Work out the finished part from the listing and answer in its coordinate system (mm). A direction names the side the tool comes from. Coordinates: 2 decimals unless noted, no trailing zeros. Loops run counter-clockwise (first coordinate to the right, second up) from the corner with the lowest first, then second, coordinate; pieces in that order, holes last. Notation, with made-up numbers: (-26, 13.5) -> (11, 13.5) arc R14 cw to (11, 28.5) -> close; hole circle Ø2 at (40.25, 76.5). An arc over 180 degrees is marked (long way). Use a Markdown table: item, result.
from build123d import *

# Parameters (mm, degrees)
F1_DEPTH = 50.8
F0_R     = 1.016
F2_DEPTH = 31.496
F3_R     = 2.159
F4_DEPTH = 20.32
F3_W     = 39.116
F3_H     = 6.35
F3_H_2   = 9.431579427
F5_DEPTH = 25.4
F6_W     = 95.504
F6_H     = 27.8849071284
F7_DEPTH = 35.56


with BuildPart() as f1:
    # F0 (on Right) → F1 (new body, symmetric)
    with BuildSketch(Plane.YZ):
        Polygon((-42.0039315899, 10.0997092374), (-35.6157857536, 10.0997092374), (8.7960684101, 10.0997092374), (6.0031614266, 16.4607279003), (-42.0039315899, 35.4997092374), (-42.0039315899, 20.2597092374), align=None)
    extrude(amount=F1_DEPTH, both=True)

    # F0 (on Right) → F2 (join, symmetric)
    with BuildSketch(Plane.YZ):
        with BuildLine():
            Line((-48.3539315899, 10.0997092374), (-42.0039315899, 10.0997092374))
            Line((-42.0039315899, 10.0997092374), (-42.0039315899, 20.2597092374))
            Line((-42.0039315899, 20.2597092374), (-48.3539315899, 20.2597092374))
            ThreePointArc((-48.3539315899, 20.2597092374), (-51.0480084262, 19.1437860737), (-52.1639315899, 16.4497092374))
            Line((-52.1639315899, 16.4497092374), (-52.1639315899, 13.9097092374))
            ThreePointArc((-52.1639315899, 13.9097092374), (-51.0480084262, 11.215632401), (-48.3539315899, 10.0997092374))
        make_face()
        with Locations((-47.7287806571, 15.2929993346)):
            Circle(F0_R, mode=Mode.SUBTRACT)
    extrude(amount=F2_DEPTH, both=True)

    # F3 (on face) → F4 (join)
    with BuildSketch(Plane.XY.offset(20.2597092374)):
        with Locations((-24.638, -45.1789315899)):
            Circle(F3_R)
        with Locations((24.638, -45.1789315899)):
            Circle(F3_R)
    extrude(amount=F4_DEPTH)

    # F3 (on face) → F5 (cut)
    with BuildSketch(Plane.XY.offset(20.2597092374)):
        with Locations((0, -45.1789315899)):
            Rectangle(F3_W, F3_H)
        with Locations((0, -53.0697213034)):
            Rectangle(F3_W, F3_H_2)
    extrude(amount=-F5_DEPTH, mode=Mode.SUBTRACT)

    # F6 (on Front) → F7 (cut, symmetric)
    with BuildSketch(Plane.XZ):
        with Locations((0, 27.0901628016)):
            Rectangle(F6_W, F6_H)
    extrude(amount=F7_DEPTH, both=True, mode=Mode.SUBTRACT)


solid = f1.part
Q1. Section D-D on x = -24 is taken. Determine the outline of the cut face in (y, z), and give its area (3 significant figures).
Solved:
| item | result |
|---|---|
| outline | (-52.16, 13.91) arc R3.81 ccw to (-48.35, 10.1) -> (8.8, 10.1) -> (7.46, 13.15) -> (-35.56, 13.15) -> (-35.56, 32.94) -> (-42, 35.5) -> (-42, 20.26) -> (-43.12, 20.26) -> (-43.12, 40.58) -> (-47.24, 40.58) -> (-47.24, 20.26) -> (-48.35, 20.26) arc R3.81 ccw to (-52.16, 16.45) -> close; hole circle Ø2.03 at (-47.73, 15.29) |
| area | 466 mm² |
Q2. Consider line 1 (X direction, y = -14.5, z = 14); line 2 (Y direction, x = -22, z = 16.5); line 3 (Z direction, x = -43.5, y = -33.5). Determine where each line is inside the solid, lowest interval first. Write a range as [from, to].
Solved:
| item | result |
|---|---|
| line 1 | [-50.8, -47.75], [47.75, 50.8] |
| line 2 | [-52.16, -35.56] |
| line 3 | [10.1, 13.15] |
Q3. Section A-A on z = 24 is taken. Determine the outline of the cut face in (x, y), and give its area (3 significant figures).
Solved:
| item | result |
|---|---|
| outline | (-50.8, -42) -> (50.8, -42) -> (50.8, -13.01) -> (47.75, -13.01) -> (47.75, -35.56) -> (-47.75, -35.56) -> (-47.75, -13.01) -> (-50.8, -13.01) -> close; circle Ø4.32 at (-24.64, -45.18); circle Ø4.32 at (24.64, -45.18) |
| area | 821 mm² |
Q4. Given pin 1 Ø3 at (x, y) = (-28.5, -46) entering from +Z; pin 2 Ø10 at (x, y) = (31, -15) entering from +Z; pin 3 Ø12 at (x, z) = (-9.5, 23.5) entering from -Y, each flat-ended and moving along its own axis, determine where each tip first touches the part or whether it passes through.
Solved:
| item | result |
|---|---|
| pin 1 | z = 20.26 |
| pin 2 | z = 13.15 |
| pin 3 | y = -42 |
Q5. Determine the mould class of faces 1 (the flat face through (50.8, -23, 20)), 2 (the cylindrical face through (25.44, -46.79, 14.9)), 3 (the flat face through (-3.5, -35.7, 33)) for opening direction Y: pulls with the +Y half, pulls with the -Y half, needs draft (parallel to the pull), parting line crosses it, or undercut.
Solved:
| item | result |
|---|---|
| face 1 | needs draft |
| face 2 | undercut |
| face 3 | pulls with the +Y half |
Q6. For faces 4 (the flat face through (19.558, -46, 15)), 5 (the flat face through (-1, -35.56, 23)), 6 (the flat face through (-27, -44, 20.26)), 7 (the flat face through (0.71, 8.35, 11.12)), determine the directions among +Z, -Z, +X, -X, +Y, -Y from which every point of the face is accessible in a straight line to the end or side of a thin tool.
Solved:
| item | result |
|---|---|
| face 4 | +Z, -Z, -Y |
| face 5 | +Z, +Y |
| face 6 | +Z |
| face 7 | +Z, +X, -X, +Y |
Q7. Section C-C on y = 0 is taken. Determine the outline of the cut face in (x, z), and give its area (3 significant figures).
Solved:
| item | result |
|---|---|
| outline | (-50.8, 10.1) -> (50.8, 10.1) -> (50.8, 18.84) -> (47.75, 18.84) -> (47.75, 13.15) -> (-47.75, 13.15) -> (-47.75, 18.84) -> (-50.8, 18.84) -> close |
| area | 344 mm² |
Q8. Section B-B on x = -2.5 is taken. Determine the outline of the cut face in (y, z).
Solved:
| item | result |
|---|---|
| outline | (-42, 10.1) -> (8.8, 10.1) -> (7.46, 13.15) -> (-35.56, 13.15) -> (-35.56, 32.94) -> (-42, 35.5) -> close |
